Input: part model. Units: mm. Frame: model coordinates. A direction names the side the tool comes from. Round coordinates to 2 decimals unless told otherwise and drop trailing zeros. Use CSV: the item, a comma, the result in double quotes.
```python
from build123d import *

# Parameters (mm, degrees)
F0_W     = 10
F0_H     = 1200
F1_DEPTH = 100
F3_DEPTH = 1700


with BuildPart() as f1:
    # F0 (on Right) → F1 (new body)
    with BuildSketch(Plane.YZ):
        with Locations((5, 600)):
            Rectangle(F0_W, F0_H)
    extrude(amount=F1_DEPTH)

    # F2 (on Right) → F3 (join)
    with BuildSketch(Plane.YZ):
        Polygon((0, 24.353822), (0, 49.894088), (-45.105246, 33.477121), (-36.896762, 10.924499), align=None)
        Polygon((-45.105245, 93.47712), (-36.896762, 70.924497), (1e-06, 84.35382), (1e-06, 109.894087), align=None)
        Polygon((-45.105244, 153.477119), (-36.896761, 130.924496), (2e-06, 144.353819), (2e-06, 169.894086), align=None)
        Polygon((-45.105243, 213.477117), (-36.89676, 190.924495), (3e-06, 204.353818), (3e-06, 229.894084), align=None)
        Polygon((-45.105242, 273.477116), (-36.896759, 250.924493), (3e-06, 264.353816), (3e-06, 289.894083), align=None)
        Polygon((-45.105241, 393.477113), (-36.896757, 370.924491), (5e-06, 384.353814), (5e-06, 409.89408), align=None)
        Polygon((-45.10524, 453.477112), (-36.896757, 430.924489), (6e-06, 444.353812), (6e-06, 469.894079), align=None)
        Polygon((-45.105242, 333.477115), (-36.896758, 310.924492), (4e-06, 324.353815), (4e-06, 349.894082), align=None)
        Polygon((-45.105239, 513.477111), (-36.896756, 490.924488), (7e-06, 504.353811), (7e-06, 529.894078), align=None)
        Polygon((-45.105237, 633.477108), (-36.896754, 610.924485), (8e-06, 624.353808), (8e-06, 649.894075), align=None)
        Polygon((-45.105238, 573.477109), (-36.896755, 550.924487), (8e-06, 564.35381), (8e-06, 589.894076), align=None)
        Polygon((-45.105237, 693.477107), (-36.896753, 670.924484), (9e-06, 684.353807), (9e-06, 709.894074), align=None)
        Polygon((-45.105236, 753.477105), (-36.896752, 730.924482), (1e-05, 744.353806), (1e-05, 769.894072), align=None)
        Polygon((-45.105233, 933.477101), (-36.89675, 910.924478), (1.3e-05, 924.353802), (1.3e-05, 949.894068), align=None)
        Polygon((-45.105235, 813.477104), (-36.896752, 790.924481), (1.1e-05, 804.353804), (1.1e-05, 829.894071), align=None)
        Polygon((-45.105234, 873.477103), (-36.896751, 850.92448), (1.2e-05, 864.353803), (1.2e-05, 889.89407), align=None)
        Polygon((-45.10523, 1173.477096), (-36.896747, 1150.924473), (1.6e-05, 1164.353796), (1.6e-05, 1189.894063), align=None)
        Polygon((-45.105231, 1113.477097), (-36.896747, 1090.924474), (1.5e-05, 1104.353798), (1.5e-05, 1129.894064), align=None)
        Polygon((-45.105232, 1053.477099), (-36.896748, 1030.924476), (1.4e-05, 1044.353799), (1.4e-05, 1069.894066), align=None)
        Polygon((-45.105232, 993.4771), (-36.896749, 970.924477), (1.3e-05, 984.3538), (1.3e-05, 1009.894067), align=None)
    extrude(amount=F3_DEPTH)


solid = f1.part
```
Item 1: Line query: line 1 (X direction, y = 5, z = 583); line 2 (Y direction, x = 895, z = 692.5). Output: solid intervals per line, ascending.
Worked answers:
line 1,"x = 0 to 100"
line 2,"y = -44.75 to 0"
Item 2: Set-up query: faces 3 (the face through (1700, -23, 331)), 4 (the face through (838.1, -22.24, 821.8)). Return all of +Z, -Z, +X, -X, +Y, -Y with unobstructed straight access to the full face (end or side cutting, diameter ignored); none if empty.
Worked answers:
face 3,"+Z, -Z, +X, +Y, -Y"
face 4,"+X, -X, -Y"
Item 3: Section query A-A on x = 1243.5. Give the number of separate pieces and of enclosed holes in the cut face, plus the area to 3 significant figures.
Worked answers:
separate pieces,"20"
enclosed holes,"0"
area,"20,900 mm²"
Item 4: Pull-direction query (Z, two-part tool) for faces 1 (the face through (838.1, -18.707, 677.545)), 2 (the face through (1700, -23, 391)); classes: +Z half, -Z half, draft (parallel to the pull), parting line (faces both ways), or undercut.
Worked answers:
face 1,"undercut"
face 2,"draft"
Item 5: First-contact query: pin 1 Ø20.5 at (x, z) = (586.5, 453.5) entering from +Y; pin 2 Ø1 at (x, y) = (507, -6.5) entering from +Z; pin 3 Ø1.5 at (x, y) = (439.5, -3.5) entering from -Z. Flat tips, straight axial feed; report the tip coordinate or a pass-through.
Worked answers:
pin 1,"stops at y = 0"
pin 2,"stops at z = 1187.71"
pin 3,"stops at z = 22.81"
